Work out the finished part from the listing and answer in its coordinate system (mm). A direction names the side the tool comes from. Give positions to 0.01 mm unless a question says otherwise; leave off trailing zeros. Loops run counter-clockwise (first coordinate to the right, second up) from the corner with the lowest first, then second, coordinate; pieces in that order, holes last. Notation, with made-up numbers: (30.5, 49.5) -> (62.5, 49.5) arc R16 ccw to (62.5, 70.5) -> close; hole circle Ø10 at (-30, -17.5). An arc over 180 degrees is marked (long way). Answer as CSV lines item,"result". Start each with the question number.
1. Find the intervals of material crossed by line 1 along X through (y, z) = (8, 12.5); line 2 along X through (y, z) = (4, -23); line 3 along Y through (x, z) = (640.5, 11.5), in increasing order.
2. Determine the mould class of faces 1 (the face through (865, -7, 0)), 2 (the face through (507, -21.334, -21)), 3 (the face through (507, 27, -65)) for opening direction Z: +Z half, -Z half, draft (parallel to the pull), parting line (faces both ways), or undercut.
3. Flat-ended cylindrical pins translate along their axes: pin 1 Ø12 at (x, z) = (766.5, -45) entering from +Y; pin 2 Ø3 at (x, z) = (389.5, -53.5) entering from +Y; pin 3 Ø1.5 at (x, z) = (333, -16.5) entering from +Y. Find the tip coordinate at first contact, or state that the pin passes through.
4. A tool of negligible diameter and unlimited length cuts with its end or side. For faces 4 (the face through (125.384, 38, -21)), 5 (the face through (850.357, -3.451, -3.252)), 6 (the face through (204, 0, -16)), from which of +Z, -Z, +X, -X, +Y, -Y can it reach the whole face along a straight path? Write none if from no direction.
5. Find section D-D, the plane x = 583. Give the vertices of the cut face in (y, z).
6. Find section C-C, the plane z = 8. Give the vertices of the cut face in (x, y).
7. Find section B-B, the plane x = 865. Give the vertices of the cut face in (y, z).
8. Find section A-A, the plane y = 44.5. Give the vertices of the cut face in (x, z).
from build123d import *

# Parameters (mm, degrees)
CUT_EXTRUDE7_DEPTH               = 1010.950493836
CUT_EXTRUDE7_DEPTH_BACK          = 1010.950493836
SKETCH13_W                       = 48.176434887
SKETCH13_H                       = 155.804640487
SKETCH4_W                        = 600
SKETCH4_H                        = 44.158972604
CUT_EXTRUDE2_DEPTH               = 1010.950493836
SKETCH7_W                        = 159.807953253
SKETCH7_H                        = 69.49104999
BOSS_EXTRUDE7_DEPTH              = 5
FILLET5_R                        = 10
F_5_8_0_625_DIAMETER_HOLE1_D     = 15.875
F_5_8_0_625_DIAMETER_HOLE1_DEPTH = 30
F_5_8_0_625_DIAMETER_HOLE1_TIP   = 4.769331164
BOSS_EXTRUDE8_DEPTH              = 10
BOSS_EXTRUDE8_DEPTH_BACK         = 10
SKETCH16_W                       = 57.403477863
SKETCH16_H                       = 23.203595883
SKETCH17_W                       = 38.256761469
SKETCH17_H                       = 12.64819079
BOSS_EXTRUDE9_DEPTH              = 10
SKETCH18_W                       = 120
SKETCH18_H                       = 104.74536306
CUT_EXTRUDE8_DEPTH               = 161
FILLET6_R                        = 10
SKETCH19_R                       = 15
CUT_EXTRUDE9_DEPTH               = 7
CUT_EXTRUDE11_DEPTH              = 1010.950493856
CUT_EXTRUDE11_DEPTH_BACK         = 1010.950493856
SKETCH22_W                       = 1481.455902665
SKETCH22_H                       = 524.99926461
SKETCH22_W_2                     = 774.615564444
SKETCH22_H_2                     = 130
SKETCH23_W                       = 1033.221047575
SKETCH23_H                       = 313.410359552
SKETCH23_W_2                     = 790.959514037
SKETCH23_H_2                     = 163.499719248
CUT_EXTRUDE12_DEPTH              = 915.822387207
CUT_EXTRUDE13_DEPTH              = 908.868382599
CUT_EXTRUDE13_DEPTH_BACK         = 908.868382599
SKETCH24_W                       = 774.615564444
SKETCH24_H                       = 42.920513698


# Read off the part's stored shape, not the designer's step: Revolve1
with BuildPart() as part:
    # Revolve1 outline → Revolve1 (revolve)
    with BuildSketch(Plane.YX):
        with BuildLine():
            Line((0, 1000), (0, 0))
            ThreePointArc((0, 0), (70.710678154, 29.289321917), (100, 100.0000001))
            Line((100, 100.0000001), (100, 899.9999999))
            ThreePointArc((100, 899.9999999), (70.710678154, 970.710678083), (0, 1000))
        make_face()
    revolve(axis=Axis((0, 0, 0), (1, 0, 0)))

    # Sketch13 → Cut-Extrude7 (cut, two sides: drawn at the far end of the back side and taken through both)
    with BuildSketch(Plane(origin=(0, 0, 0), x_dir=(1, 0, 0), z_dir=(0, 1, 0)).offset(-CUT_EXTRUDE7_DEPTH_BACK)):
        with Locations((5.911782557, -3.075091589)):
            Rectangle(SKETCH13_W, SKETCH13_H)
    extrude(amount=CUT_EXTRUDE7_DEPTH + CUT_EXTRUDE7_DEPTH_BACK, mode=Mode.SUBTRACT)

    # Sketch4 → Cut-Extrude2 (cut, through all)
    with BuildSketch(Plane(origin=(0, 0, 0), x_dir=(1, 0, 0), z_dir=(0, 1, 0))):
        with Locations((595, 0)):
            Rectangle(SKETCH4_W, SKETCH4_H)
    extrude(amount=CUT_EXTRUDE2_DEPTH, mode=Mode.SUBTRACT)

    # Sketch7 → Boss-Extrude7 (add)
    with BuildSketch(Plane(origin=(0, 0, 0), x_dir=(1, 0, 0), z_dir=(0, 1, 0))):
        with Locations((745.885521462, -1.405844332)):
            Rectangle(SKETCH7_W, SKETCH7_H)
    extrude(amount=-BOSS_EXTRUDE7_DEPTH)

    # Fillet5
    fillet5_edges = [part.edges().sort_by_distance(p)[0] for p in [
        (30, -71.414284286, 0),
    ]]
    fillet(fillet5_edges, radius=FILLET5_R)

    # 5/8 (0.625) Diameter Hole1
    with Locations(Plane.ZY.offset(-30)):
        with Locations((0, 0)):
            Hole(F_5_8_0_625_DIAMETER_HOLE1_D / 2, depth=F_5_8_0_625_DIAMETER_HOLE1_DEPTH)
            with Locations((0, 0, -(F_5_8_0_625_DIAMETER_HOLE1_DEPTH + F_5_8_0_625_DIAMETER_HOLE1_TIP / 2))):  # 118° drill point
                Cone(0, F_5_8_0_625_DIAMETER_HOLE1_D / 2, F_5_8_0_625_DIAMETER_HOLE1_TIP, mode=Mode.SUBTRACT)

    # Sketch16 → Boss-Extrude8 (add, two sides: drawn at the far end of the back side and taken through both)
    with BuildSketch(Plane.XY.offset(-BOSS_EXTRUDE8_DEPTH_BACK)):
        with Locations((738.294537666, -11.601797942)):
            Rectangle(SKETCH16_W, SKETCH16_H)
    extrude(amount=BOSS_EXTRUDE8_DEPTH + BOSS_EXTRUDE8_DEPTH_BACK)

    # Sketch17 → Boss-Extrude9 (add)
    with BuildSketch(Plane.XY.offset(-22.079486302)):
        with Locations((787.071835847, 6.324095395)):
            Rectangle(SKETCH17_W, SKETCH17_H)
    extrude(amount=-BOSS_EXTRUDE9_DEPTH)

    # Sketch18 → Cut-Extrude8 (cut)
    with BuildSketch(Plane(origin=(0, 0, 0), x_dir=(1, 0, 0), z_dir=(0, 1, 0))):
        with Locations((204.992275313, 0)):
            Rectangle(SKETCH18_W, SKETCH18_H)
    extrude(amount=CUT_EXTRUDE8_DEPTH, mode=Mode.SUBTRACT)

    # Fillet6
    fillet6_edges = [part.edges().sort_by_distance(p)[0] for p in [
        (144.992275313, 42.594313674, -52.37268153),
        (144.992275313, 42.594313674, 52.37268153),
        (264.992275313, 42.594313674, 52.37268153),
        (264.992275313, 42.594313674, -52.37268153),
    ]]
    fillet(fillet6_edges, radius=FILLET6_R)

    # Sketch19 → Cut-Extrude9 (cut)
    with BuildSketch(Plane(origin=(0, 0, 0), x_dir=(1, 0, 0), z_dir=(0, 1, 0))):
        with Locations(Location((865, 0, 0), (0, 0, 270))):
            Circle(SKETCH19_R)
    extrude(amount=-CUT_EXTRUDE9_DEPTH, mode=Mode.SUBTRACT)

    # Sketch22 → Cut-Extrude11 (cut, two sides: drawn at the far end of the back side and taken through both)
    with BuildSketch(Plane(origin=(0, 0, 0), x_dir=(1, 0, 0), z_dir=(0, 1, 0)).offset(-CUT_EXTRUDE11_DEPTH_BACK)):
        with Locations((406.155110175, 0)):
            Rectangle(SKETCH22_W, SKETCH22_H)
        with Locations((512.692217778, 0)):
            Rectangle(SKETCH22_W_2, SKETCH22_H_2, mode=Mode.SUBTRACT)
    extrude(amount=CUT_EXTRUDE11_DEPTH + CUT_EXTRUDE11_DEPTH_BACK, mode=Mode.SUBTRACT)

    # Sketch23 → Cut-Extrude12 (cut, through all)
    with BuildSketch(Plane.XY.offset(65)):
        with Locations((481.89787613, -1.932796335)):
            Rectangle(SKETCH23_W, SKETCH23_H)
        with Locations((520.864192575, 60.415600646)):
            Rectangle(SKETCH23_W_2, SKETCH23_H_2, mode=Mode.SUBTRACT)
    extrude(amount=-CUT_EXTRUDE12_DEPTH, mode=Mode.SUBTRACT)

    # Sketch24 → Cut-Extrude13 (cut, two sides: drawn at the far end of the back side and taken through both)
    with BuildSketch(Plane(origin=(0, 0, 0), x_dir=(1, 0, 0), z_dir=(0, 1, 0)).offset(-CUT_EXTRUDE13_DEPTH_BACK)):
        with Locations((512.692217778, -43.539743151)):
            Rectangle(SKETCH24_W, SKETCH24_H)
    extrude(amount=CUT_EXTRUDE13_DEPTH + CUT_EXTRUDE13_DEPTH_BACK, mode=Mode.SUBTRACT)


solid = part.part
Resolved:
1,line 1,"x = 125.38 to 144.99, 264.99 to 295, 895 to 900"
1,line 2,"x = 125.38 to 144.99, 264.99 to 900"
1,line 3,"y = -21.33 to 0"
2,face 1,"undercut"
2,face 2,"draft"
2,face 3,"-Z half"
3,pin 1,"stops at y = 92.08"
3,pin 2,"stops at y = 85.42"
3,pin 3,"stops at y = 0"
4,face 4,"+Z, -Z, -X, +Y, -Y"
4,face 5,"+Y"
4,face 6,"+Z, +Y"
5,outline,"(-21.33, -65) -> (75.99, -65) arc R100 ccw to (97.53, -22.08) -> (0, -22.08) -> (0, 22.08) -> (-21.33, 22.08) -> close"
6,outline,"(125.38, -21.33) -> (900, -21.33) -> (900, 99.68) -> (895, 99.68) -> (895, 0) -> (877.69, 0) -> (877.69, -7) -> (852.31, -7) -> (852.31, 0) -> (295, 0) -> (295, 99.68) -> (264.99, 99.68) -> (264.99, 0) -> (144.99, 0) -> (144.99, 99.68) -> (125.38, 99.68) -> close"
7,outline,"(-21.33, -65) -> (75.99, -65) arc R100 ccw to (97.53, -22.08) -> (0, -22.08) -> (0, -15) -> (-7, -15) -> (-7, 15) -> (0, 15) -> (0, 22.08) -> (-21.33, 22.08) -> close"
8,outline,"(125.38, -65) -> (900, -65) -> (900, 22.08) -> (895, 22.08) -> (895, -22.08) -> (295, -22.08) -> (295, 22.08) -> (264.99, 22.08) -> (264.99, -42.37) arc R10 cw to (254.99, -52.37) -> (154.99, -52.37) arc R10 cw to (144.99, -42.37) -> (144.99, 22.08) -> (125.38, 22.08) -> close"
